Check sheet for the modelled part. Datum: model origin and axes. Units: mm. A direction names the side the tool comes from. Give positions to 0.01 mm unless a question says otherwise; leave off trailing zeros. Order: outer loops, then holes, each group sorted by start corner. A loop starts at its lowest first (then second) coordinate and runs counter-clockwise, first axis right, second up.
from build123d import *

# Parameters (mm, degrees)
EXTRUDE_1_DEPTH     = 2
SKETCH_2_R          = 4
EXTRUDE_2_DEPTH     = 6
SKETCH_3_R          = 3
CUT_EXTRUDE_1_DEPTH = 4
CHAMFER_1_SIZE      = 1


with BuildPart() as part:
    # Эскиз1 → Бобышка-Вытянуть1 (new body)
    with BuildSketch(Plane.XY):
        with BuildLine():
            Line((-3.5, 5), (3.5, 5))
            ThreePointArc((3.5, 5), (8.5, 0), (3.5, -5))
            Line((3.5, -5), (-3.5, -5))
            ThreePointArc((-3.5, -5), (-8.5, 0), (-3.5, 5))
        make_face()
    extrude(amount=EXTRUDE_1_DEPTH)

    # Эскиз2 → Бобышка-Вытянуть2 (add)
    with BuildSketch(Plane.XY.offset(2)):
        Circle(SKETCH_2_R)
    extrude(amount=EXTRUDE_2_DEPTH)

    # Эскиз3 → Вырез-Вытянуть1 (cut)
    with BuildSketch(Plane(origin=(0, 0, 0), x_dir=(-1, 0, 0), z_dir=(0, 0, -1))):
        Circle(SKETCH_3_R)
    extrude(amount=-CUT_EXTRUDE_1_DEPTH, mode=Mode.SUBTRACT)

    # Фаска1
    chamfer_1_edges = [part.edges().sort_by_distance(p)[0] for p in [
        (-4, 0, 8),
    ]]
    chamfer(chamfer_1_edges, length=CHAMFER_1_SIZE)


solid = part.part
1) Depth check by flat-ended pin: pin 1 Ø2 at (x, z) = (1, 5) entering from +Y; pin 2 Ø2 at (x, z) = (-4.5, 2.5) entering from -Y; pin 3 Ø2 at (x, y) = (4, -4) entering from -Z; pin 4 Ø1 at (x, z) = (3.5, 7) entering from -Y. Enter the tip coordinate at first touch or a pass-through.
Recorded:
pin 1: stops at y = 4
pin 2: stops at y = -5
pin 3: stops at z = 0
pin 4: stops at y = -2.65
2) Material ranges on L1, parallel to Z at x = 5.75, y = -3.75; L2, parallel to X at y = -2, z = 1.5; L3, parallel to X at y = 1.25, z = 1, recorded low to high.
Recorded:
L1: z = 0 to 2
L2: x = -8.08 to -2.24, 2.24 to 8.08
L3: x = -8.34 to -2.73, 2.73 to 8.34
3) Section check D-D, the plane z = 6.25. Record the cut outline in (x, y), then the cut area to 3 significant figures.
Recorded:
outline: circle Ø8 at (0, 0)
area: 50.3 mm2
4) Set-up check for faces 1 (the face through (-0.867, -3.905, 4.465)), 2 (the face through (8.5, 0.1, 1)): record each of +Z, -Z, +X, -X, +Y, -Y from which the full face is reachable in a straight line by a thin tool's end or side.
Recorded:
face 1: +Z
face 2: +Z, -Z, +X
5) Section check C-C, the plane z = 7.5. Record the cut outline in (x, y), then the cut area to 3 significant figures.
Recorded:
outline: circle Ø7 at (0, 0)
area: 38.5 mm2
6) Section check A-A, the plane y = 0. Record the cut outline in (x, z).
Recorded:
outline: (-8.5, 0) - (-3, 0) - (-3, 4) - (3, 4) - (3, 0) - (8.5, 0) - (8.5, 2) - (4, 2) - (4, 7) - (3, 8) - (-3, 8) - (-4, 7) - (-4, 2) - (-8.5, 2) - close
7) Draft check along Y on faces 3 (the face through (-8.5, -0.1, 1)), 4 (the face through (3, 0, 2)), 5 (the face through (0, -5, 1)), 6 (the face through (0, 0, 4)). Enter one of: +Y half, -Y half, draft (parallel to the pull), parting line (faces both ways), or undercut.
Recorded:
face 3: parting line
face 4: undercut
face 5: -Y half
face 6: undercut
8) Section check B-B, the plane x = 0. Record the cut outline in (y, z).
Recorded:
outline: (-5, 0) - (-3, 0) - (-3, 4) - (3, 4) - (3, 0) - (5, 0) - (5, 2) - (4, 2) - (4, 7) - (3, 8) - (-3, 8) - (-4, 7) - (-4, 2) - (-5, 2) - close
